Geometry check sheet. Reference: drawing and pictorial views, mm from the part's lowest x, y, z. A direction names the side the tool comes from. Round coordinates to 2 decimals unless told otherwise and drop trailing zeros. Write each loop counter-clockwise with the first axis right and the second up, starting at its lowest first coordinate (ties: lowest second). Pieces come first, ordered by that corner, then holes.
Item 1: Section check C-C, the plane z = 9. Record the cut outline in (x, y), plus the area to 3 significant figures.
Item 2: Section check A-A, the plane z = 19.05. Record the cut outline in (x, y).
Item 3: Set-up check for the marked faces 1 and 2: record each of +Z, -Z, +X, -X, +Y, -Y from which the full face is reachable in a straight line by a thin tool's end or side.
Item 4: Material ranges on line 1 along X through (y, z) = (27.5, 17); line 2 along Y through (x, z) = (5.5, 22), recorded low to high.
Item 5: Section check B-B, the plane y = 17. Record the cut outline in (x, z), plus the area to 3 significant figures.
Item 6: Depth check by flat-ended pin: pin 1 (1.5 mm diameter, centred on y = 13, z = 23, fed in from -X). Enter the tip coordinate at first touch or a pass-through.
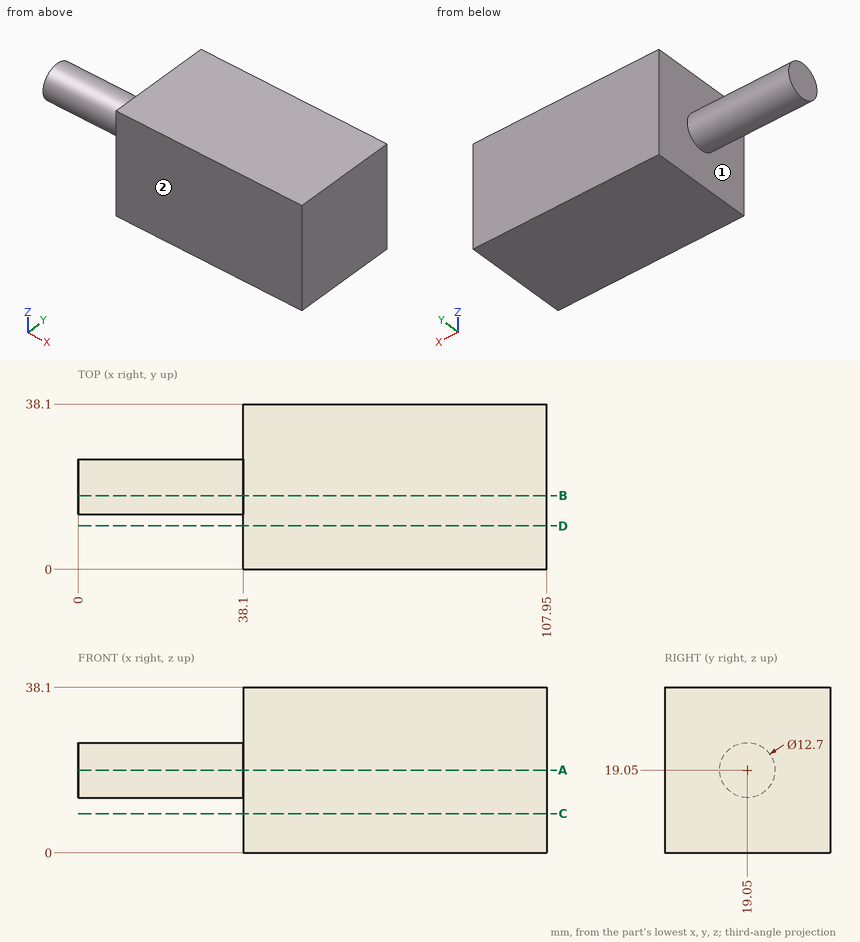
Values found:
1. outline: (38.1, 0) - (107.95, 0) - (107.95, 38.1) - (38.1, 38.1) - close
1. area: 2,660 mm2
2. outline: (0, 12.7) - (38.1, 12.7) - (38.1, 0) - (107.95, 0) - (107.95, 38.1) - (38.1, 38.1) - (38.1, 25.4) - (0, 25.4) - close
3. face 1: -X
3. face 2: +Z, -Z, +X, -X, -Y
4. line 1: x = 38.1 to 107.95
4. line 2: y = 13.43 to 24.67
5. outline: (0, 13.04) - (38.1, 13.04) - (38.1, 0) - (107.95, 0) - (107.95, 38.1) - (38.1, 38.1) - (38.1, 25.06) - (0, 25.06) - close
5. area: 3,120 mm2
6. pin 1: stops at x = 38.1
